```python
from build123d import *

# Parameters (mm, degrees)
SKETCH_1_W          = 26.4
SKETCH_1_H          = 15.7
EXTRUDE_1_DEPTH     = 31.5
SKETCH_2_W          = 3.8
SKETCH_2_H          = 4
EXTRUDE_2_DEPTH     = 4.4
SKETCH_3_W          = 3.8
SKETCH_3_H          = 4
EXTRUDE_3_DEPTH     = 4.4
SKETCH_4_R          = 0.975
CUT_EXTRUDE_1_DEPTH = 37.92739498
FILLET_1_R          = 0.8


with BuildPart() as part:
    # ｽｹｯﾁ1 → ﾎﾞｽ - 押し出し1 (new body)
    with BuildSketch(Plane(origin=(0, 0, 0), x_dir=(1, 0, 0), z_dir=(0, 1, 0))):
        Rectangle(SKETCH_1_W, SKETCH_1_H)
    extrude(amount=EXTRUDE_1_DEPTH)

    # ｽｹｯﾁ2 → ﾎﾞｽ - 押し出し2 (add)
    with BuildSketch(Plane(origin=(13.2, 0, 0), x_dir=(0, 0, -1), z_dir=(1, 0, 0))):
        with Locations((-5.95, 2)):
            Rectangle(SKETCH_2_W, SKETCH_2_H)
        with Locations((5.95, 2)):
            Rectangle(SKETCH_2_W, SKETCH_2_H)
    extrude(amount=EXTRUDE_2_DEPTH)

    # ｽｹｯﾁ3 → ﾎﾞｽ - 押し出し3 (add)
    with BuildSketch(Plane.ZY.offset(13.2)):
        with Locations((5.95, 2)):
            Rectangle(SKETCH_3_W, SKETCH_3_H)
        with Locations((-5.95, 2)):
            Rectangle(SKETCH_3_W, SKETCH_3_H)
    extrude(amount=EXTRUDE_3_DEPTH)

    # ｽｹｯﾁ4 → ｶｯﾄ - 押し出し1 (cut, through all)
    with BuildSketch(Plane.XZ):
        with Locations(Location((4, 0, 0), (0, 0, 270))):
            Circle(SKETCH_4_R)
        with Locations(Location((-4, 0, 0), (0, 0, 270))):
            Circle(SKETCH_4_R)
    extrude(amount=-CUT_EXTRUDE_1_DEPTH, mode=Mode.SUBTRACT)

    # ﾌｨﾚｯﾄ1
    fillet_1_edges = [part.edges().sort_by_distance(p)[0] for p in [
        (15.4, 4, 4.05),
        (15.4, 4, -4.05),
        (-15.4, 4, 4.05),
        (-15.4, 4, -4.05),
    ]]
    fillet(fillet_1_edges, radius=FILLET_1_R)


solid = part.part
```
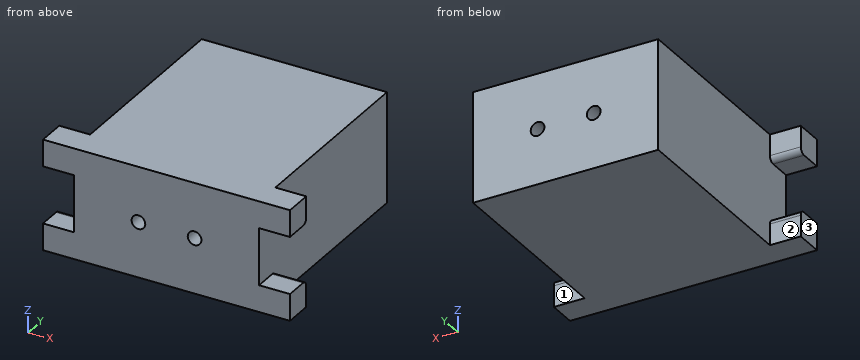
Geometry: final body of the model. Coordinates: model frame, mm. Face numbers are marked on the shaded views. A direction names the side the tool comes from. Round coordinates to 2 decimals unless told otherwise and drop trailing zeros. Write each loop counter-clockwise with the first axis right and the second up, starting at its lowest first coordinate (ties: lowest second). Pieces come first, ordered by that corner, then holes. Notation, with made-up numbers: M -37.75,7 L -23.75,7 A6 cw -23.75,15 Z; hole C 13.5,-34 d1. An arc over 180 degrees is marked long. Answer in a Markdown table with one row per item. Add a question column.
(1) Cut plane D-D, the plane z = 2. Return the cut outline in (x, y).
(2) Cut plane A-A, the plane x = -4. Return the cut outline in (y, z) (3 decimals), then the cut area to 3 significant figures.
(3) Cut plane B-B, the plane y = 6. Return the cut outline in (x, z) (3 decimals), then the cut area to 3 significant figures.
(4) Contact query for flat-ended pins moving along their axis: pin 1 (3.5 mm diameter, centred on x = -15.5, z = -7, fed in from +Y); pin 2 (8 mm diameter, centred on y = 11, z = -2, fed in from +X); pin 3 (8 mm diameter, centred on x = -1.5, z = 2, fed in from -Y); pin 4 (4 mm diameter, centred on y = 27, z = -1, fed in from -X). Output: stop coordinate, or through.
(5) Reachability of the marked faces 1, 2 and 3 from +Z, -Z, +X, -X, +Y, -Y: full face, straight path, thin tool, end or side. Return the list, or none.
(6) Ray query, L1, parallel to X at y = 23, z = 0 (3 decimals); L2, parallel to X at y = 28.5, z = 6.75. Return the intervals inside material, ascending.
(7) Cut plane C-C, the plane z = -6.25. Return the cut outline in (x, y).
Established:
| question | item | result |
|---|---|---|
| 1 | outline | M -13.2,0 L 13.2,0 L 13.2,31.5 L -13.2,31.5 Z |
| 2 | outline | M 0,-7.85 L 31.5,-7.85 L 31.5,-0.975 L 0,-0.975 Z; M 0,0.975 L 31.5,0.975 L 31.5,7.85 L 0,7.85 Z |
| 2 | area | 433 mm² |
| 3 | outline | M -13.2,-7.85 L 13.2,-7.85 L 13.2,7.85 L -13.2,7.85 Z; hole C -4,0 d1.95; hole C 4,0 d1.95 |
| 3 | area | 409 mm² |
| 4 | pin 1 | y = 4 |
| 4 | pin 2 | x = 13.2 |
| 4 | pin 3 | y = 0 |
| 4 | pin 4 | x = -13.2 |
| 5 | face 1 | +Z, -Z, +X, +Y |
| 5 | face 2 | +Z, -Z, -X, +Y |
| 5 | face 3 | +Z, -Z, -X, +Y, -Y |
| 6 | L1 | -13.2 to -4.975, -3.025 to 3.025, 4.975 to 13.2 |
| 6 | L2 | -13.2 to 13.2 |
| 7 | outline | M -17.6,0 L 17.6,0 L 17.6,4 L 13.2,4 L 13.2,31.5 L -13.2,31.5 L -13.2,4 L -17.6,4 Z |
